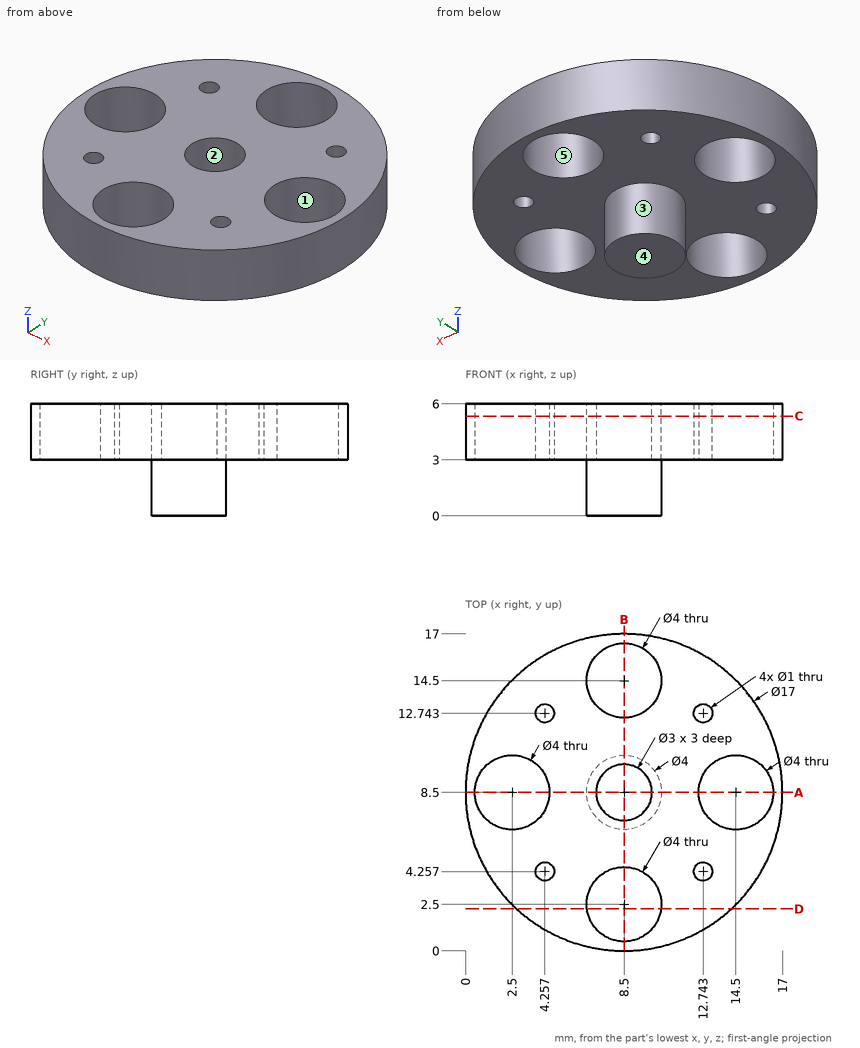
Check sheet for the drawn part. Datum: minimum x, y, z corner. Units: mm. A direction names the side the tool comes from. Round coordinates to 2 decimals unless told otherwise and drop trailing zeros. Order: outer loops, then holes, each group sorted by start corner. A loop starts at its lowest first (then second) coordinate and runs counter-clockwise, first axis right, second up.
(1) Access from +Z, -Z, +X, -X, +Y, -Y to the whole of each face (thin tool, end or side, straight path). Record for the marked faces 1 and 2.
(2) Cross-section at C-C, the plane z = 5.35. State how many separate pieces and enclosed holes the cut face has.
(3) Cross-section at A-A, the plane y = 8.5. Enter the section's corners in (x, z), and give its area (3 significant figures).
(4) Go/stop test with flat-tipped pins: P1, Ø3.5, axis at x = 8.5, y = 14.5, coming from the +Z side; P2, Ø2, axis at x = 5.5, z = 3, coming from the +Y side; P3, Ø2, axis at x = 13, y = 15, coming from the -Z side; P4, Ø2.5, axis at x = 8.5, y = 8.5, coming from the +Z side. Record where each tip stops, or that it passes through.
(5) Scan lines: probe 1 along Y at (x, z) = (8.5, 5.2); probe 2 along Y at (x, z) = (6.75, 3.8) (1 decimal); probe 3 along Z at (x, y) = (2, 5.25). Record each from-to range of solid material in increasing order.
(6) Draft check along Y on the marked faces 3, 4 and 5. Enter one of: pulls with the +Y half, pulls with the -Y half, needs draft (parallel to the pull), parting line crosses it, or undercut.
(7) Cross-section at D-D, the plane y = 2.25. Enter the section's corners in (x, z) (1 decimal).
Check sheet entries:
1. face 1: +Z, -Z
1. face 2: +Z
2. separate pieces: 1
2. enclosed holes: 9
3. outline: (0, 3) - (0.5, 3) - (0.5, 6) - (0, 6) - close; (4.5, 3) - (6.5, 3) - (6.5, 0) - (10.5, 0) - (10.5, 3) - (12.5, 3) - (12.5, 6) - (10, 6) - (10, 3) - (7, 3) - (7, 6) - (4.5, 6) - close; (16.5, 3) - (17, 3) - (17, 6) - (16.5, 6) - close
3. area: 30.0 mm2
4. P1: passes through
4. P2: stops at y = 16.76
4. P3: stops at z = 3
4. P4: stops at z = 3
5. probe 1: y = 0 to 0.5, 4.5 to 7, 10 to 12.5, 16.5 to 17
5. probe 2: y = 0.2 to 1.5, 3.5 to 13.5, 15.5 to 16.8
5. probe 3: z = 3 to 6
6. face 3: parting line crosses it
6. face 4: needs draft
6. face 5: undercut
7. outline: (2.7, 3) - (6.5, 3) - (6.5, 6) - (2.7, 6) - close; (10.5, 3) - (14.3, 3) - (14.3, 6) - (10.5, 6) - close
